Could you check a few things on this model? Use its own coordinates, in mm. Face numbers are marked on the shaded views. A direction names the side the tool comes from. Give positions to 0.01 mm unless a question says otherwise; leave off trailing zeros. Write each loop counter-clockwise with the first axis right and the second up, starting at its lowest first coordinate (ties: lowest second). Pieces come first, ordered by that corner, then holes. Notation, with made-up numbers: M 18,68.25 L 38,68.25 A33 ccw 38,102.25 Z; hole C 38,-25 d8. An arc over 180 degrees is marked long. Answer as a JSON object with one key per item and string values. Group by question number.
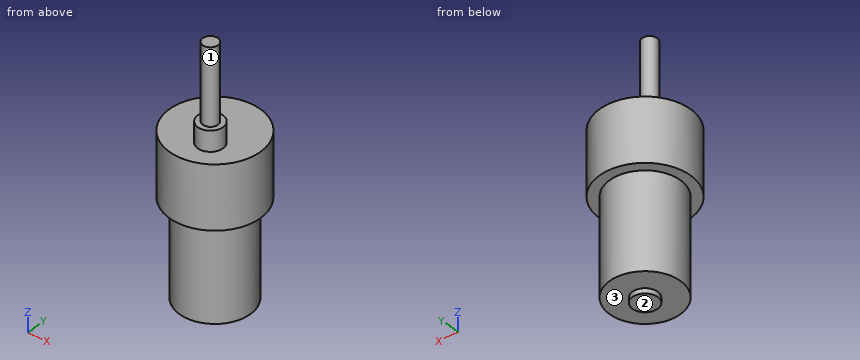
```python
from build123d import *

# Parameters (mm, degrees)
SKETCH1_R           = 18
BOSS_EXTRUDE1_DEPTH = 25
SKETCH2_R           = 14
BOSS_EXTRUDE2_DEPTH = 38
SKETCH3_R           = 5
BOSS_EXTRUDE3_DEPTH = 2
SKETCH4_R           = 5
BOSS_EXTRUDE4_DEPTH = 8
SKETCH5_R           = 3
BOSS_EXTRUDE5_DEPTH = 30


with BuildPart() as part:
    # Sketch1 → Boss-Extrude1 (new body)
    with BuildSketch(Plane.XY):
        Circle(SKETCH1_R)
    extrude(amount=BOSS_EXTRUDE1_DEPTH)

    # Sketch2 → Boss-Extrude2 (add)
    with BuildSketch(Plane(origin=(0, 0, 0), x_dir=(-1, 0, 0), z_dir=(0, 0, -1))):
        Circle(SKETCH2_R)
    extrude(amount=BOSS_EXTRUDE2_DEPTH)

    # Sketch3 → Boss-Extrude3 (add)
    with BuildSketch(Plane(origin=(0, 0, -38), x_dir=(-1, 0, 0), z_dir=(0, 0, -1))):
        Circle(SKETCH3_R)
    extrude(amount=BOSS_EXTRUDE3_DEPTH)

    # Sketch4 → Boss-Extrude4 (add)
    with BuildSketch(Plane.XY.offset(25)):
        with Locations((2.991643327, -5.770621301)):
            Circle(SKETCH4_R)
    extrude(amount=BOSS_EXTRUDE4_DEPTH)

    # Sketch5 → Boss-Extrude5 (add)
    with BuildSketch(Plane.XY.offset(33)):
        with Locations((2.991643327, -5.770621301)):
            Circle(SKETCH5_R)
    extrude(amount=BOSS_EXTRUDE5_DEPTH)


solid = part.part
```
1) I'm going to push flat-ended pins straight in: pin 1 (3 mm diameter, centred on y = -12.5, z = -3, fed in from -X); pin 2 (3 mm diameter, centred on x = 3.5, z = 34, fed in from +Y); pin 3 (8 mm diameter, centred on x = -2, y = 4.5, fed in from +Z); pin 4 (8 mm diameter, centred on x = -7.5, z = 32.5, fed in from -Y). Where does each tip first touch, or does it pass through?
2) For the marked faces 1, 2 and 3, which set-ups out of +Z, -Z, +X, -X, +Y, -Y let a thin tool reach every point of the face, with its end or its side?
3) If we section it at C-C, the plane z = -32: List the corners of the cut face in (x, y) for me, plus the area to 3 significant figures.
4) Please list where these lines run through material, in increasing order: line 1 along Z through (x, y) = (-3, -6.5); line 2 along Z through (x, y) = (-13, -9); line 3 along X through (y, z) = (-11, -21). Write a range as from..to.
5) If we section it at B-B, the plane y = 12.5: List the corners of the cut face in (x, z) for me, plus the area to 3 significant figures.
6) If we section it at A-A, the plane x = -8: List the corners of the cut face in (y, z) for me, plus the area to 3 significant figures.
7) If we section it at D-D, the plane z = 21: List the corners of the cut face in (x, y) for me.
Taken from the geometry:
{
 "1": {"pin 1": "x = -8.66", "pin 2": "y = -0.77", "pin 3": "z = 25", "pin 4": "through"},
 "2": {"face 1": "+Z", "face 2": "-Z, +X, -X, +Y, -Y", "face 3": "-Z"},
 "3": {"outline": "C 0,0 d28", "area": "616 mm²"},
 "4": {"line 1": "-38..25", "line 2": "0..25", "line 3": "-8.66..8.66"},
 "5": {"outline": "M -12.95,0 L -6.3,0 L -6.3,-38 L 6.3,-38 L 6.3,0 L 12.95,0 L 12.95,25 L -12.95,25 Z", "area": "1,130 mm²"},
 "6": {"outline": "M -16.12,0 L -11.49,0 L -11.49,-38 L 11.49,-38 L 11.49,0 L 16.12,0 L 16.12,25 L -16.12,25 Z", "area": "1,680 mm²"},
 "7": {"outline": "C 0,0 d36"}
}
